Autodesk Inventor part; units mm, degrees
ref_plane "YZ Plane" through (0, 0, 0) normal (1, 0, 0) x (0, 1, 0)
ref_plane "XZ Plane" through (0, 0, 0) normal (0, 1, 0) x (-1, 0, 0)
ref_plane "XY Plane" through (0, 0, 0) normal (0, 0, 1) x (1, 0, 0)
sketch "Sketch1" plane through (0, 0, 0) normal (1, 0, 0) x (0, 1, 0)
  line L0 (82.3549, 41.969) -> (-47.6451, 41.969)
  line L1 (-47.6451, 41.969) -> (-47.6451, -28.031)
  line L2 (-47.6451, -28.031) -> (82.3549, -28.031)
  line L3 (82.3549, -28.031) -> (82.3549, 41.969)
  point P0 (0, 0)
  dimension "d0" = 130
  dimension "d1" = 70
extrude "Extrusion1" add sketch "Sketch1" along normal blind 5
sketch "Sketch13" plane through (5, 0, 0) normal (1, 0, 0) x (0, 0, -1)
  line L0 (-41.969, -47.6451) -> (28.031, -47.6451)
  line L1 (28.031, 82.3549) -> (-41.969, 82.3549)
  line L2 (28.031, -47.6451) -> (26.531, -47.6451)
  line L3 (26.531, -47.6451) -> (26.531, 82.3549)
  line L4 (26.531, 82.3549) -> (28.031, 82.3549)
  line L5 (28.031, 82.3549) -> (28.031, -47.6451)
  line L6 (-41.969, 82.3549) -> (-41.969, -47.6451)
  line L7 (28.031, 82.3549) -> (-41.969, 82.3549)
  line L8 (-41.969, -47.6451) -> (-40.469, -47.6451)
  line L9 (-40.469, -47.6451) -> (-40.469, 82.3549)
  line L10 (-40.469, 82.3549) -> (-41.969, 82.3549)
  line L11 (-41.969, 82.3549) -> (-41.969, -47.6451)
  line L12 (28.031, -47.6451) -> (-41.969, -47.6451)
  line L13 (-41.969, -47.6451) -> (-41.969, -45.6451)
  line L14 (-41.969, -45.6451) -> (28.031, -45.6451)
  line L15 (28.031, -45.6451) -> (28.031, -47.6451)
  point P0 (0, 0)
  point P1 (10.031, 62.3549)
  point P2 (-5.969, 62.3549)
  point P3 (26.531, -45.6451)
  point P4 (-40.469, -45.6451)
  point P5 (18.031, 62.3549)
  dimension "d42" = 1.5
  dimension "d43" = 1.5
  dimension "d44" = 2
extrude "Extrusion7" add sketch "Sketch13" along normal blind 0.01 contours L6 L14 L9 L0 | L9 L14 L3 L0 | L6 L1 L9 L14 | L3 L14 L5 L0 | L3 L1 L5 L14
sketch "Sketch18" plane through (5, 0, 0) normal (1, 0, 0) x (0, 0, -1)
  line L0 (-10.769, 82.3549) -> (-2.569, 82.3549)
  line L1 (-2.569, 82.3549) -> (-2.2688, 82.3549)
  line L2 (-10.769, 82.3549) -> (-11.069, 82.3549)
  line L3 (-11.069, 82.3549) -> (-11.069, 78.5449)
  line L4 (-2.2688, 82.3549) -> (-2.2688, 78.5449)
  line L5 (-2.2688, 78.5449) -> (4.6812, 78.5449)
  line L6 (-11.069, 78.5449) -> (-18.019, 78.5449)
  line L7 (-18.019, 78.5449) -> (-18.019, 73.5449)
  line L8 (4.6812, 78.5449) -> (4.6812, 73.5449)
  line L9 (-18.019, 73.5449) -> (-7.137, 73.5449)
  line L10 (-7.137, 73.5449) -> (4.6812, 73.5449)
  line L11 (-2.2688, 82.3549) -> (-11.069, 82.3549)
  line L12 (26.531, 82.3549) -> (26.531, -45.6451)
  point P0 (0, 0)
  point P1 (4.531, 82.3549)
  point P2 (-3.669, 82.3549)
  point P3 (11.531, 82.3549)
  dimension "d78" = 7.4
  dimension "d79" = 3.81
  dimension "d81" = 3.81
  dimension "d83" = 6.95
  dimension "d85" = 6.95
  dimension "d86" = 5
  dimension "d87" = 5
  dimension "d88" = 8.8002
  dimension "d91" = 11.8183
  dimension "d92" = 10.8819
extrude "Extrusion10" cut sketch "Sketch18" against normal blind 7.9375
properties part number "baseplateinverseproto 1"
Design review of the part built by this model. Coordinates are the model's own, in mm. A direction names the side the tool comes from. Round coordinates to 2 decimals unless told otherwise and drop trailing zeros. Order: outer loops, then holes, each group sorted by start corner. A loop starts at its lowest first (then second) coordinate and runs counter-clockwise, first axis right, second up. Notation, with made-up numbers: M 49.5,27.25 L 63.5,27.25 A23 ccw 63.5,39.25 Z; hole C 59.25,-7 d6. An arc over 180 degrees is marked long. Answer as CSV lines item,"result". Start each with the question number.
1) For pin 1 Ø3 at (y, z) = (2, -10.5) entering from -X, flat-tipped, find the tip position at first contact; note if it passes through.
2) The part is to be moulded in two halves that separate along Y. For faces 1 (the face through (2, -47.645, 7)), 2 (the face through (2, 82.355, -13)), 3 (the face through (5, 17, 7)), 4 (the face through (3, 73.545, 7)), say which applies: +Y half, -Y half, draft (parallel to the pull), parting line (faces both ways), or undercut.
3) Add section B-B (x = 2.85). Give the boundary of the cut face in (y, z).
4) Wall thickness on line 1 along Y through (x, z) = (3.2, 17); line 2 along Y through (x, z) = (2.6, 6); line 3 along X through (y, z) = (6, 33): over which ranges is each line inside the solid? List them lowest first. Write a range as [from, to].
5) Tool access review of faces 5 (the face through (2, 82.355, 26)), 6 (the face through (3, 80, 2.269)), 7 (the face through (3, 78.545, -1)): name each direction out of +Z, -Z, +X, -X, +Y, -Y from which nothing blocks a thin tool from reaching the whole face with its end or side.
Resolved:
1,pin 1,"x = 0"
2,face 1,"-Y half"
2,face 2,"+Y half"
2,face 3,"draft"
2,face 4,"undercut"
3,outline,"M -47.65,-28.03 L 82.35,-28.03 L 82.35,2.27 L 78.54,2.27 L 78.54,-4.68 L 73.54,-4.68 L 73.54,18.02 L 78.54,18.02 L 78.54,11.07 L 82.35,11.07 L 82.35,41.97 L -47.65,41.97 Z"
4,line 1,"[-47.65, 73.54], [78.54, 82.35]"
4,line 2,"[-47.65, 73.54]"
4,line 3,"[0, 5]"
5,face 5,"+Z, -Z, +X, -X, +Y"
5,face 6,"+X, -X, +Y"
5,face 7,"+X, -X"
